```python
from build123d import *

# Parameters (mm, degrees)
F0_R     = 9.44458633
F1_DEPTH = 25.4
F2_D     = 15.24
F3_D     = 15.24
F4_D     = 15.24


with BuildPart() as f1:
    # F0 (on Front) → F1 (new body)
    with BuildSketch(Plane.XZ):
        with BuildLine():
            Line((44.0184436738, 12.1698062867), (-43.5005836189, 12.1698062867))
            ThreePointArc((-43.5005836189, 12.1698062867), (-55.4114580154, 0.2589318901), (-43.5005836189, -11.6519425064))
            Line((-43.5005836189, -11.6519425064), (44.0184436738, -11.6519425064))
            ThreePointArc((44.0184436738, -11.6519425064), (55.9293180704, 0.2589318901), (44.0184436738, 12.1698062867))
        make_face()
        with Locations((-36.7683507502, 0)):
            Circle(F0_R, mode=Mode.SUBTRACT)
        Circle(F0_R, mode=Mode.SUBTRACT)
        with Locations((37.8040745854, 0)):
            Circle(F0_R, mode=Mode.SUBTRACT)
        with Locations((-36.7683507502, 0)):
            Circle(F0_R)
        Circle(F0_R)
        with Locations((37.8040745854, 0)):
            Circle(F0_R)
    extrude(amount=F1_DEPTH)

    # F2 (through all)
    with Locations(Plane(origin=(0, 0, 0), x_dir=(1, 0, 0), z_dir=(0, 1, 0))):
        with Locations((-36.7683507502, 0)):
            Hole(F2_D / 2)

    # F3 (through all)
    with Locations(Plane(origin=(0, 0, 0), x_dir=(1, 0, 0), z_dir=(0, 1, 0))):
        with Locations((0, 0)):
            Hole(F3_D / 2)

    # F4 (through all)
    with Locations(Plane(origin=(0, 0, 0), x_dir=(1, 0, 0), z_dir=(0, 1, 0))):
        with Locations((37.8040745854, 0)):
            Hole(F4_D / 2)


solid = f1.part
```
Work out the finished part from the listing and answer in its coordinate system (mm). Give positions to 0.01 mm unless a question says otherwise; leave off trailing zeros. Order: outer loops, then holes, each group sorted by start corner. A loop starts at its lowest first (then second) coordinate and runs counter-clockwise, first axis right, second up. Notation, with made-up numbers: (39.5, 88) - (59.5, 88) arc R18 cw to (59.5, 122) - close; hole circle Ø3 at (22, -8.5). An arc over 180 degrees is marked (long way). One line per item, written item: value. Start each with the question number.
1. Section B-B, the plane y = -8.25 is taken. Write down the section's boundary in (x, z).
2. Section A-A, the plane x = 0 is taken. Write down the section's boundary in (y, z).
3. Each of these flat-tipped pins is pushed along its axis until it touches: pin 1 Ø6 at (x, z) = (-40, -3) entering from +Y; pin 2 Ø10 at (y, z) = (-15.5, -8.5) entering from -X; pin 3 Ø12 at (y, z) = (-9.5, 7) entering from +X; pin 4 Ø10 at (x, y) = (45, -14) entering from -Z. Where does it stop, or does it pass through?
4. Section C-C, the plane z = 0 is taken. Write down the section's boundary in (x, y), then the cut area to 3 significant figures.
5. For a pull along X with two mould halves and no side action, classify faces 1 (the face through (-1, -25.4, 8)), 2 (the face through (30.536, -12.878, -2.289)), 3 (the face through (-55.41, -12.52, 0.52)), 4 (the face through (55.926, -12.522, -0.003)) as released by +X, released by -X, zero draft, split by the parting line, or undercut.
6. Section D-D, the plane x = -32.5 is taken. Write down the section's boundary in (y, z).
7. Consider line 1 (X direction, y = -10.5, z = -0.25); line 2 (Z direction, x = 0, y = -8.25); line 3 (X direction, y = -8.25, z = 4). Determine where each line is inside the solid, lowest interval first.
Filled sheet:
1. outline: (-43.5, -11.65) - (44.02, -11.65) arc R11.91 ccw to (44.02, 12.17) - (-43.5, 12.17) arc R11.91 ccw to start; hole circle Ø15.24 at (-36.77, 0); hole circle Ø15.24 at (0, 0); hole circle Ø15.24 at (37.8, 0)
2. outline: (-25.4, -11.65) - (0, -11.65) - (0, -7.62) - (-25.4, -7.62) - close; (-25.4, 7.62) - (0, 7.62) - (0, 12.17) - (-25.4, 12.17) - close
3. pin 1: through
3. pin 2: x = -54.8
3. pin 3: x = 55.91
3. pin 4: z = -11.65
4. outline: (-55.41, -25.4) - (-44.39, -25.4) - (-44.39, 0) - (-55.41, 0) - close; (-29.15, -25.4) - (-7.62, -25.4) - (-7.62, 0) - (-29.15, 0) - close; (7.62, -25.4) - (30.18, -25.4) - (30.18, 0) - (7.62, 0) - close; (45.42, -25.4) - (55.93, -25.4) - (55.93, 0) - (45.42, 0) - close
4. area: 1,670 mm²
5. face 1: zero draft
5. face 2: undercut
5. face 3: released by -X
5. face 4: released by +X
6. outline: (-25.4, -11.65) - (0, -11.65) - (0, -6.31) - (-25.4, -6.31) - close; (-25.4, 6.31) - (0, 6.31) - (0, 12.17) - (-25.4, 12.17) - close
7. line 1: -55.4 to -44.38, -29.15 to -7.62, 7.62 to 30.19, 45.42 to 55.92
7. line 2: -11.65 to -7.62, 7.62 to 12.17
7. line 3: -54.81 to -43.25, -30.28 to -6.49, 6.49 to 31.32, 44.29 to 55.33
